Source: CAD feature listing. Evaluate the final solid. Frame: model axes, mm. A direction names the side the tool comes from. Give positions to 0.01 mm unless a question says otherwise; leave off trailing zeros. Order: outer loops, then holes, each group sorted by start corner. A loop starts at its lowest first (then second) coordinate and runs counter-clockwise, first axis right, second up. Notation, with made-up numbers: M -4.75,13 L 24.25,13 A22 ccw 24.25,36 Z; hole C -11.5,-35 d8. An arc over 180 degrees is marked long. One line per question, with ' | ' between items. Start each with the question number.
from build123d import *

# Parameters (mm, degrees)
SKETCH3_W          = 1
SKETCH3_H          = 14
CUT_EXTRUDE2_DEPTH = 15


with BuildPart() as part:
    # Sketch1 → Revolve1 (revolve)
    with BuildSketch(Plane(origin=(0, 0, 0), x_dir=(0, 0, -1), z_dir=(1, 0, 0)), mode=Mode.PRIVATE) as revolve1_sk:
        Polygon((-5.5, 6), (5.5, 6), (5.5, 9.9), (5, 10), (5.5, 10.1), (5.5, 12.5), (4, 14), (-4, 14), (-5.5, 12.5), (-5.5, 10.1), (-5, 10), (-5.5, 9.9), align=None)
    revolve(revolve1_sk.sketch.rotate(Axis((0, 0, 10.112306333), (0, 0, -1)), 90), axis=Axis((0, 0, 10.112306333), (0, 0, -1)))

    # Sketch3 → Cut-Extrude2 (cut, symmetric)
    with BuildSketch(Plane.XY):
        with Locations((0, 7)):
            Rectangle(SKETCH3_W, SKETCH3_H)
    extrude(amount=CUT_EXTRUDE2_DEPTH, both=True, mode=Mode.SUBTRACT)


solid = part.part
Item 1: Cut plane B-B on z = -2.75. Return the cut outline in (x, y), and give its area (3 significant figures).
Item 2: Pin query (flat end, axial travel): pin 1 Ø1 at (y, z) = (3, 4) entering from +X (3 decimals); pin 2 Ø4 at (y, z) = (11.5, -2.5) entering from +X; pin 3 Ø7 at (x, y) = (0, 0) entering from +Z; pin 4 Ø8 at (x, y) = (0, 3) entering from +Z. Return the tip coordinate at first contact, or that it passes through.
Item 3: Cut plane A-A on x = 0. Return the cut outline in (y, z).
Item 4: Reachability of faces 3 (the flat face through (9, 5, 5.5)), 4 (the flat face through (0.5, 10, 0)) from +Z, -Z, +X, -X, +Y, -Y: full face, straight path, thin tool, end or side. Return the list, or none.
Item 5: Mould query, pull axis Y, two halves, no side actions, for faces 1 (the flat face through (4, -5, 5.5)), 2 (the cylindrical face through (0, -6, 0)). Classes: pulls with the +Y half, pulls with the -Y half, needs draft (parallel to the pull), parting line crosses it, or undercut.
Item 6: Line query: line 1 (Y direction, x = 0, z = 2); line 2 (X direction, y = 2.5, z = -0.75); line 3 (X direction, y = -3.25, z = -2.5). Output: solid intervals per line, ascending.
Item 7: Cut plane C-C on z = 4.5. Return the cut outline in (x, y).
Results are:
1) outline: M -0.5,5.98 L -0.5,13.99 A14 ccw long 0.5,13.99 L 0.5,5.98 A6 cw long Z | area: 495 mm2
2) pin 1: stops at x = 13.775 | pin 2: stops at x = 10.28 | pin 3: passes through | pin 4: stops at z = 5.5
3) outline: M -14,-4 L -12.5,-5.5 L -10.1,-5.5 L -10,-5 L -9.9,-5.5 L -6,-5.5 L -6,5.5 L -9.9,5.5 L -10,5 L -10.1,5.5 L -12.5,5.5 L -14,4 Z
4) face 3: +Z, +X, -X, +Y, -Y | face 4: +Z, -Z, +Y
5) face 1: needs draft | face 2: undercut
6) line 1: y = -14 to -6 | line 2: x = -13.77 to -5.45, 5.45 to 13.77 | line 3: x = -13.62 to -5.04, 5.04 to 13.62
7) outline: M -0.5,5.98 L -0.5,13.49 A13.5 ccw long 0.5,13.49 L 0.5,5.98 A6 cw long Z
